from build123d import *

# Parameters (mm, degrees)
SKETCH1_W           = 66
SKETCH1_H           = 30
BOSS_EXTRUDE1_DEPTH = 31
SKETCH2_W           = 64
SKETCH2_H           = 26
CUT_EXTRUDE1_DEPTH  = 25
SKETCH3_R           = 1
BOSS_EXTRUDE2_DEPTH = 30
SKETCH4_W           = 6
SKETCH4_H           = 6
CUT_EXTRUDE2_DEPTH  = 8.25
SKETCH5_W           = 6
SKETCH5_H           = 6
CUT_EXTRUDE3_DEPTH  = 8.25
SKETCH6_W           = 0.5
SKETCH6_H           = 8.25
CUT_EXTRUDE4_DEPTH  = 31
CUT_EXTRUDE5_DEPTH  = 2


with BuildPart() as part:
    # Sketch1 → Boss-Extrude1 (new body)
    with BuildSketch(Plane(origin=(0, 0, 0), x_dir=(1, 0, 0), z_dir=(0, 1, 0))):
        Rectangle(SKETCH1_W, SKETCH1_H)
    extrude(amount=BOSS_EXTRUDE1_DEPTH)

    # Sketch2 → Cut-Extrude1 (cut)
    with BuildSketch(Plane(origin=(0, 31, 0), x_dir=(1, 0, 0), z_dir=(0, 1, 0))):
        with Locations((-1, 0)):
            Rectangle(SKETCH2_W, SKETCH2_H)
    extrude(amount=-CUT_EXTRUDE1_DEPTH, mode=Mode.SUBTRACT)

    # Sketch3 → Boss-Extrude2 (add)
    with BuildSketch(Plane.XY.offset(15)):
        with BuildLine():
            Line((-36, 0), (-33, 0))
            Line((-33, 0), (-33, 6))
            Line((-33, 6), (-36, 6))
            ThreePointArc((-36, 6), (-39, 3), (-36, 0))
        make_face()
        with Locations((-36, 3)):
            Circle(SKETCH3_R, mode=Mode.SUBTRACT)
    extrude(amount=-BOSS_EXTRUDE2_DEPTH)

    # Sketch4 → Cut-Extrude2 (cut)
    with BuildSketch(Plane.XY.offset(15)):
        with Locations((-36, 3)):
            Rectangle(SKETCH4_W, SKETCH4_H)
    extrude(amount=-CUT_EXTRUDE2_DEPTH, mode=Mode.SUBTRACT)

    # Sketch5 → Cut-Extrude3 (cut)
    with BuildSketch(Plane(origin=(0, 0, -15), x_dir=(-1, 0, 0), z_dir=(0, 0, -1))):
        with Locations((36, 3)):
            Rectangle(SKETCH5_W, SKETCH5_H)
    extrude(amount=-CUT_EXTRUDE3_DEPTH, mode=Mode.SUBTRACT)

    # Sketch6 → Cut-Extrude4 (cut)
    with BuildSketch(Plane.XZ):
        with Locations((-32.75, -10.875)):
            Rectangle(SKETCH6_W, SKETCH6_H)
        with Locations((-32.75, 10.875)):
            Rectangle(SKETCH6_W, SKETCH6_H)
    extrude(amount=-CUT_EXTRUDE4_DEPTH, mode=Mode.SUBTRACT)

    # Sketch7 → Cut-Extrude5 (cut)
    with BuildSketch(Plane(origin=(33, 0, 0), x_dir=(0, 0, -1), z_dir=(1, 0, 0))):
        with BuildLine():
            Line((12, 19), (12, 31))
            Line((12, 31), (-12, 31))
            Line((-12, 31), (-12, 19))
            ThreePointArc((-12, 19), (0, 7), (12, 19))
        make_face()
    extrude(amount=-CUT_EXTRUDE5_DEPTH, mode=Mode.SUBTRACT)


solid = part.part
Here's how the part is built. I have some questions about the finished solid (model axes, mm). A direction names the side the tool comes from. Round coordinates to 2 decimals unless told otherwise and drop trailing zeros. Order: outer loops, then holes, each group sorted by start corner. A loop starts at its lowest first (then second) coordinate and runs counter-clockwise, first axis right, second up. Notation, with made-up numbers: (80, -32.75) -> (98, -32.75) arc R15 ccw to (98, -8.75) -> close; hole circle Ø9 at (29, 45.5). An arc over 180 degrees is marked (long way). Return JSON: item names as keys, results as strings.
Q1. If we section it at B-B on z = 0: List the corners of the cut face in (x, y) for me.
Filled sheet:
{"outline": "(-36, 0) -> (33, 0) -> (33, 7) -> (31, 7) -> (31, 6) -> (-36, 6) arc R3 ccw to start; hole circle Ø2 at (-36, 3)"}
Q2. If we section it at C-C on x = -6: List the corners of the cut face in (y, z) for me.
Filled sheet:
{"outline": "(0, -15) -> (31, -15) -> (31, -13) -> (6, -13) -> (6, 13) -> (31, 13) -> (31, 15) -> (0, 15) -> close"}
Q3. For pin 1 Ø5 at (x, z) = (11, 3) entering from +Y; pin 2 Ø5 at (x, y) = (-36.5, 2.5) entering from +Z; pin 3 Ø9 at (y, z) = (22, -11) entering from -X, each with a flat end and sliding along its axis, tell me the tip position at first contact or that it passes through.
Filled sheet:
{"pin 1": "stops at y = 6", "pin 2": "stops at z = 6.75", "pin 3": "stops at x = -32.5"}
Q4. Which directions (+Z, -Z, +X, -X, +Y, -Y) give clear straight access to the entire face, cutting with the end or side of a thin tool? Please do faces 5 (the flat face through (32, 25, -12)), 6 (the flat face through (31, 6.5, 0.1)), 7 (the flat face through (-32.5, 8, 14)), 8 (the flat face through (-32.5, 8, -14)).
Filled sheet:
{"face 5": "+X, -X, +Y", "face 6": "-X, +Y", "face 7": "+Z, -X, +Y, -Y", "face 8": "-Z, -X, +Y, -Y"}
Q5. If we mould it in two halves opening along Z, with no side actions, what happens to faces 1 (the flat face through (0, 31, 14)), 2 (the flat face through (-35, 2, 6.75)), 3 (the flat face through (-1, 19, 13)), 4 (the flat face through (0, 16, -15))? For each: released by +Z, released by -Z, zero draft, split by the parting line, or undercut.
Filled sheet:
{"face 1": "zero draft", "face 2": "released by +Z", "face 3": "undercut", "face 4": "released by -Z"}
Q6. I need wall thicknesses on line 1 along Z through (x, y) = (-12, 28.5); line 2 along Y through (x, z) = (-36, 0); line 3 along Y through (x, z) = (-12.5, -3.5). Which ranges of each line are inside material? Lowest first, please. Write a range as from..to.
Filled sheet:
{"line 1": "z = -15..-13, 13..15", "line 2": "y = 0..2, 4..6", "line 3": "y = 0..6"}
Q7. If we section it at A-A on y = 28: List the corners of the cut face in (x, z) for me, plus the area to 3 significant figures.
Filled sheet:
{"outline": "(-32.5, -15) -> (33, -15) -> (33, -12) -> (31, -12) -> (31, -13) -> (-32.5, -13) -> close; (-32.5, 13) -> (31, 13) -> (31, 12) -> (33, 12) -> (33, 15) -> (-32.5, 15) -> close", "area": "266 mm^2"}
Q8. If we section it at D-D on z = 3.75: List the corners of the cut face in (x, y) for me.
Filled sheet:
{"outline": "(-36, 0) -> (33, 0) -> (33, 7.6) -> (31, 7.6) -> (31, 6) -> (-36, 6) arc R3 ccw to start; hole circle Ø2 at (-36, 3)"}
